Here's the drawing with two shaded views (mm, measured from the low corner). I have some questions. Round coordinates to 2 decimals unless told otherwise and drop trailing zeros. Loops run counter-clockwise (first coordinate to the right, second up) from the corner with the lowest first, then second, coordinate; pieces in that order, holes last. Notation, with made-up numbers: M 40.25,57.25 L 48.25,57.25 A23 ccw 48.25,84.25 Z; hole C 48.5,0.25 d1. An arc over 180 degrees is marked long. Answer as CSV lines item,"result".
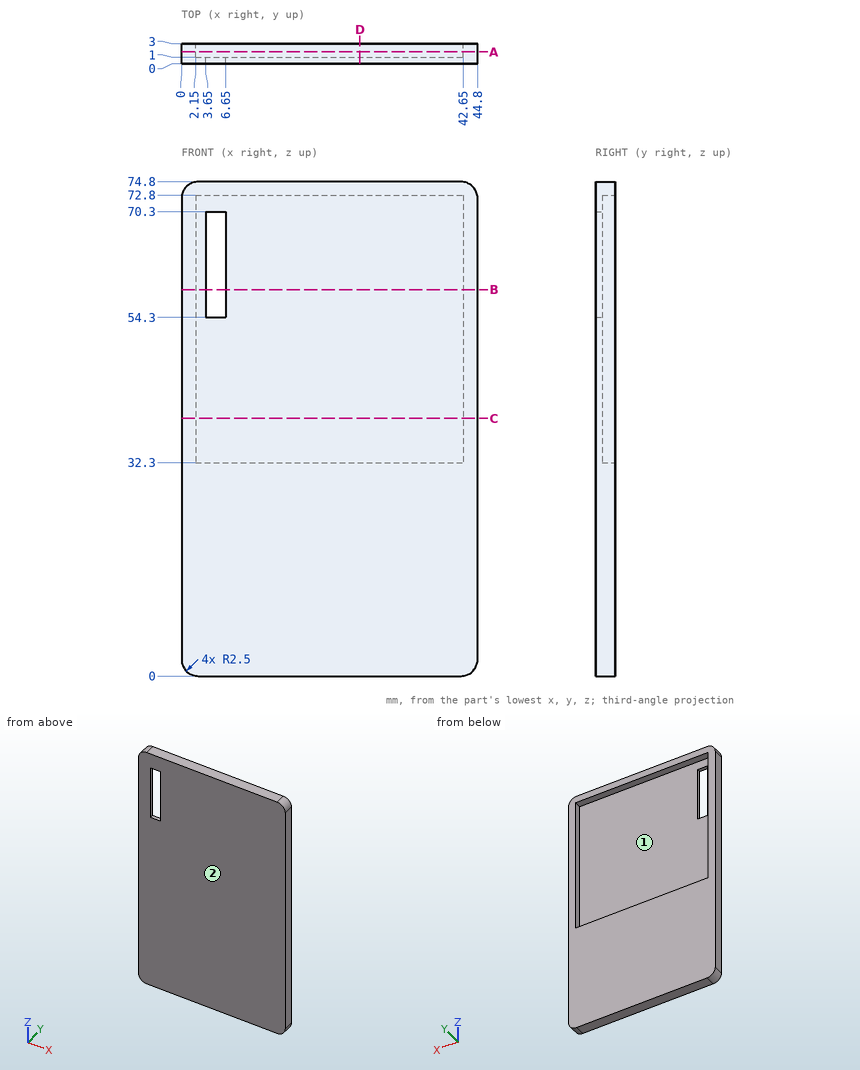
1. I want a section at A-A, the plane y = 1.8. Please give me the cut outline in (x, z), and give its area (3 significant figures).
Evaluation:
outline,"M 0,2.5 A2.5 ccw 2.5,0 L 42.3,0 A2.5 ccw 44.8,2.5 L 44.8,72.3 A2.5 ccw 42.3,74.8 L 2.5,74.8 A2.5 ccw 0,72.3 Z; hole M 2.15,32.3 L 42.65,32.3 L 42.65,72.8 L 2.15,72.8 Z"
area,"1,710 mm²"
2. I want a section at D-D, the plane x = 27. Please give me the cut outline in (y, z).
Evaluation:
outline,"M 0,0 L 3,0 L 3,32.3 L 1,32.3 L 1,72.8 L 3,72.8 L 3,74.8 L 0,74.8 Z"
3. I want a section at B-B, the plane z = 58.5. Please give me the cut outline in (x, y), and give its area (3 significant figures).
Evaluation:
outline,"M 0,0 L 3.65,0 L 3.65,1 L 2.15,1 L 2.15,3 L 0,3 Z; M 6.65,0 L 44.8,0 L 44.8,3 L 42.65,3 L 42.65,1 L 6.65,1 Z"
area,"50.4 mm²"
4. I want a section at C-C, the plane z = 39. Please give me the cut outline in (x, y).
Evaluation:
outline,"M 0,0 L 44.8,0 L 44.8,3 L 42.65,3 L 42.65,1 L 2.15,1 L 2.15,3 L 0,3 Z"
5. For P1, Ø10, axis at x = 25.5, z = 65.5, coming from the +Y side, with a flat end and sliding along its axis, tell me the tip position at first contact or that it passes through.
Evaluation:
P1,"stops at y = 1"
6. We'd pull the mould along X, two halves only. Please class the marked faces 1 and 2: pulls with the +X half, pulls with the -X half, needs draft (parallel to the pull), parting line crosses it, or undercut.
Evaluation:
face 1,"undercut"
face 2,"needs draft"
7. If I drill on line 1 (Z direction, x = 31, y = 1.1); line 2 (X direction, y = 2.15, z = 55); line 3 (Z direction, x = 4.5, y = 0.9), over which ranges is the centre line in solid material (lowest first)? Write a range as [from, to].
Evaluation:
line 1,"z = [0, 32.3], [72.8, 74.8]"
line 2,"x = [0, 2.15], [42.65, 44.8]"
line 3,"z = [0, 54.3], [70.3, 74.8]"
